```python
from build123d import *

# Parameters (mm, degrees)
SKETCH_1_W      = 80
SKETCH_1_H      = 80
SKETCH_1_R      = 1.9
SKETCH_1_R_2    = 2
SKETCH_1_R_3    = 20
EXTRUDE_1_DEPTH = 5
FILLET_5_R      = 10


with BuildPart() as part:
    # Эскиз1 → Бобышка-Вытянуть1 (new body)
    with BuildSketch(Plane(origin=(0, 0, 0), x_dir=(1, 0, 0), z_dir=(0, 1, 0))):
        Rectangle(SKETCH_1_W, SKETCH_1_H)
        with Locations(Location((20.859650045, 20.859650045, 0), (0, 0, 270))):
            Circle(SKETCH_1_R, mode=Mode.SUBTRACT)
        with Locations(Location((20.859650045, -20.859650045, 0), (0, 0, 270))):
            Circle(SKETCH_1_R, mode=Mode.SUBTRACT)
        with Locations(Location((-20.859650045, -20.859650045, 0), (0, 0, 270))):
            Circle(SKETCH_1_R, mode=Mode.SUBTRACT)
        with Locations(Location((-20.859650045, 20.859650045, 0), (0, 0, 270))):
            Circle(SKETCH_1_R, mode=Mode.SUBTRACT)
        with Locations(Location((-33, 33, 0), (0, 0, 270))):
            Circle(SKETCH_1_R_2, mode=Mode.SUBTRACT)
        with Locations(Location((33, 33, 0), (0, 0, 270))):
            Circle(SKETCH_1_R_2, mode=Mode.SUBTRACT)
        with Locations(Location((33, -33, 0), (0, 0, 270))):
            Circle(SKETCH_1_R_2, mode=Mode.SUBTRACT)
        with Locations(Location((-33, -33, 0), (0, 0, 270))):
            Circle(SKETCH_1_R_2, mode=Mode.SUBTRACT)
        with Locations(Location((0, 0, 0), (0, 0, 270))):
            Circle(SKETCH_1_R_3, mode=Mode.SUBTRACT)
        with Locations(Location((0, 29.5, 0), (0, 0, 270))):
            Circle(SKETCH_1_R_2, mode=Mode.SUBTRACT)
        with Locations(Location((29.5, 0, 0), (0, 0, 270))):
            Circle(SKETCH_1_R_2, mode=Mode.SUBTRACT)
        with Locations(Location((0, -29.5, 0), (0, 0, 270))):
            Circle(SKETCH_1_R_2, mode=Mode.SUBTRACT)
        with Locations(Location((-29.5, 0, 0), (0, 0, 270))):
            Circle(SKETCH_1_R_2, mode=Mode.SUBTRACT)
    extrude(amount=EXTRUDE_1_DEPTH)

    # Скругление5
    fillet_5_edges = [part.edges().sort_by_distance(p)[0] for p in [
        (40, 2.5, 40),
        (-40, 2.5, 40),
        (-40, 2.5, -40),
        (40, 2.5, -40),
    ]]
    fillet(fillet_5_edges, radius=FILLET_5_R)


solid = part.part
```
Check sheet for the modelled part. Datum: model origin and axes. Units: mm. Round coordinates to 2 decimals unless told otherwise and drop trailing zeros. Order: outer loops, then holes, each group sorted by start corner. A loop starts at its lowest first (then second) coordinate and runs counter-clockwise, first axis right, second up.
1) Section check D-D (z = -8). Record the boundary of the cut face in (x, y), and give its area (3 significant figures).
2) Section check A-A (z = 0). Record the boundary of the cut face in (x, y).
3) Section check B-B (x = 0). Record the boundary of the cut face in (y, z).
4) Scan lines: line 1 (Z direction, x = 22.5, y = 1.25); line 2 (X direction, y = 3.15, z = 33); line 3 (X direction, y = 2.1, z = -33.5). Record each from-to range of solid material in increasing order.
5) Mould release check, pull along X, two halves, no side actions. Record for faces 1 (the flat face through (40, 2, 0)), 2 (the flat face through (0, 2, 40)), 3 (the cylindrical face through (31.226, 2.465, -32.077)), 4 (the cylindrical face through (22.743, 2.465, 20.612)): +X half, -X half, draft (parallel to the pull), parting line (faces both ways), or undercut.
6) Section check C-C (x = 33). Record the boundary of the cut face in (y, z), and give its area (3 significant figures).
7) Go/stop test with a flat-tipped pin: pin 1 Ø2.5 at (x, z) = (20.86, -20.86) entering from +Y. Record where the tip stops, or that it passes through.
Result:
1. outline: (-40, 0) - (-18.33, 0) - (-18.33, 5) - (-40, 5) - close; (18.33, 0) - (40, 0) - (40, 5) - (18.33, 5) - close
1. area: 217 mm2
2. outline: (-40, 0) - (-31.5, 0) - (-31.5, 5) - (-40, 5) - close; (-27.5, 0) - (-20, 0) - (-20, 5) - (-27.5, 5) - close; (20, 0) - (27.5, 0) - (27.5, 5) - (20, 5) - close; (31.5, 0) - (40, 0) - (40, 5) - (31.5, 5) - close
3. outline: (0, -40) - (5, -40) - (5, -31.5) - (0, -31.5) - close; (0, -27.5) - (5, -27.5) - (5, -20) - (0, -20) - close; (0, 20) - (5, 20) - (5, 27.5) - (0, 27.5) - close; (0, 31.5) - (5, 31.5) - (5, 40) - (0, 40) - close
4. line 1: z = -40 to -21.82, -19.9 to 19.9, 21.82 to 40
4. line 2: x = -39.54 to -35, -31 to 31, 35 to 39.54
4. line 3: x = -39.37 to -34.94, -31.06 to 31.06, 34.94 to 39.37
5. face 1: +X half
5. face 2: draft
5. face 3: undercut
5. face 4: undercut
6. outline: (0, -39.54) - (5, -39.54) - (5, -35) - (0, -35) - close; (0, -31) - (5, -31) - (5, 31) - (0, 31) - close; (0, 35) - (5, 35) - (5, 39.54) - (0, 39.54) - close
6. area: 355 mm2
7. pin 1: passes through
